Print and shaded views of the part. All mm, measured from the part's lowest x, y and z. A direction names the side the tool comes from. Coordinates: 2 decimals unless noted, no trailing zeros. Loops run counter-clockwise (first coordinate to the right, second up) from the corner with the lowest first, then second, coordinate; pieces in that order, holes last. Notation, with made-up numbers: M 86,77.25 L 134,77.25 A24 ccw 134,89.25 Z; hole C 1.5,28 d10. An arc over 180 degrees is marked long. Answer as CSV lines item,"result". Start each with the question number.
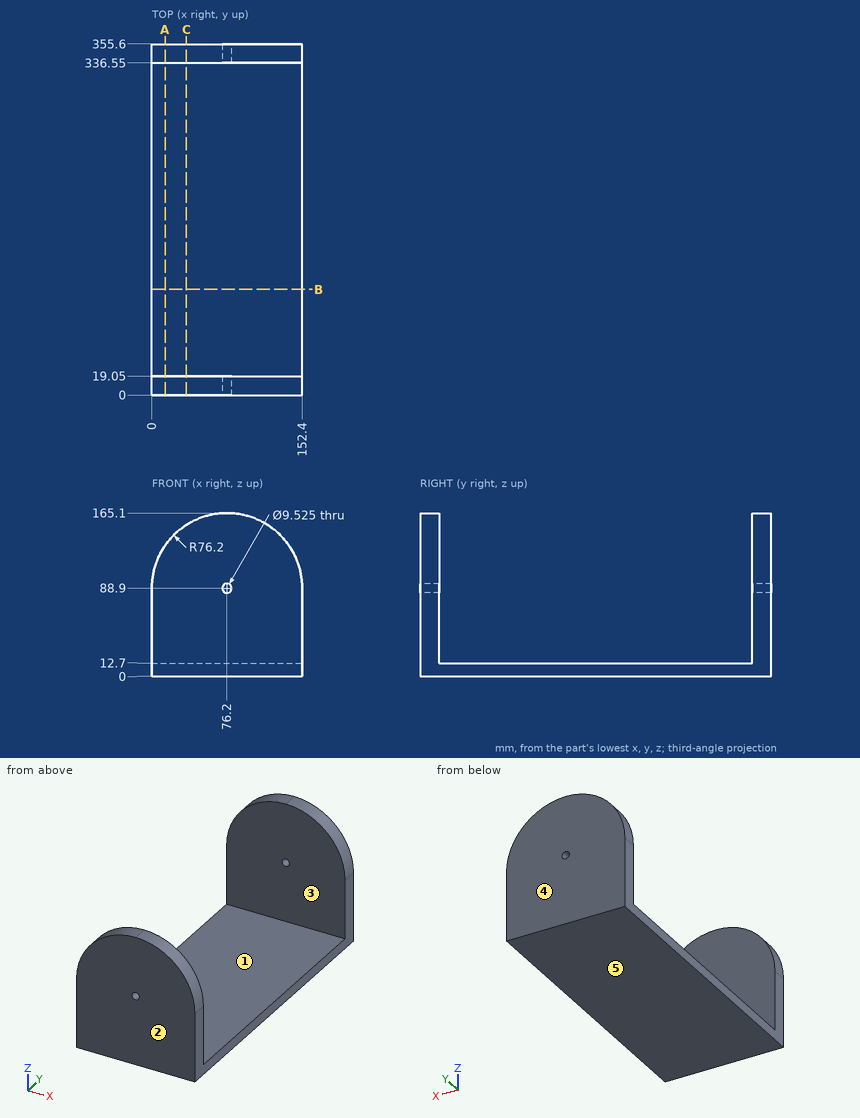
Q1. Two-plate mould, pull along Y, no slides. Class the marked faces 3, 4 and 5: +Y half, -Y half, draft (parallel to the pull), parting line (faces both ways), or undercut.
Q2. Tool access for the marked faces 1 and 2: list every direction of +Z, -Z, +X, -X, +Y, -Y with a clear straight run to the whole face (end or side of a thin tool).
Q3. Wall check: L1, parallel to Z at x = 76, y = 344; L2, parallel to Y at x = 47, z = 74.5. Give the ranges that are in metal, low to high.
Q4. Slice it at A-A, the plane x = 13.5. Write the cut outline in (y, z).
Q5. Flat gauge pin, fed straight in: P1, Ø1, axis at x = 35, y = 209.5, coming from the +Z side. Where does the tip first touch, or does it go through?
Q6. Slice it at C-C, the plane x = 35. Write the cut outline in (y, z), and give its area (3 significant figures).
Q7. Slice it at B-B, the plane y = 107. Write the cut outline in (x, z).
Solved:
1,face 3,"undercut"
1,face 4,"+Y half"
1,face 5,"draft"
2,face 1,"+Z, +X, -X"
2,face 2,"+Z, -Z, +X, -X, -Y"
3,L1,"z = 0 to 84.14, 93.66 to 165.1"
3,L2,"y = 0 to 19.05, 336.55 to 355.6"
4,outline,"M 0,0 L 355.6,0 L 355.6,132.2 L 336.55,132.2 L 336.55,12.7 L 19.05,12.7 L 19.05,132.2 L 0,132.2 Z"
5,P1,"stops at z = 12.7"
6,outline,"M 0,0 L 355.6,0 L 355.6,153 L 336.55,153 L 336.55,12.7 L 19.05,12.7 L 19.05,153 L 0,153 Z"
6,area,"9,860 mm2"
7,outline,"M 0,0 L 152.4,0 L 152.4,12.7 L 0,12.7 Z"
